Check sheet for the modelled part. Datum: model origin and axes. Units: mm. Face numbers are marked on the shaded views. A direction names the side the tool comes from. Give positions to 0.01 mm unless a question says otherwise; leave off trailing zeros. Write each loop counter-clockwise with the first axis right and the second up, starting at its lowest first coordinate (ties: lowest second). Pieces come first, ordered by that corner, then holes. Notation, with made-up numbers: (85, 63.25) -> (113, 63.25) arc R24 cw to (113, 88.25) -> close; hole circle Ø8 at (60.5, -9). An arc over 180 degrees is marked (long way). Answer as a JSON object with one key per item and string values.
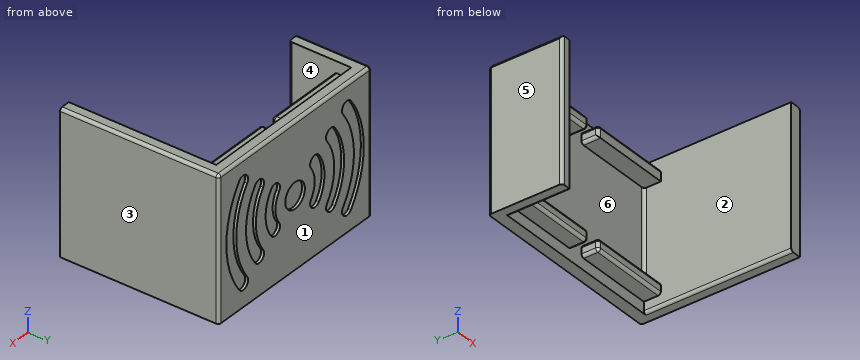
from build123d import *

# Parameters (mm, degrees)
SKETCH1_W           = 35
SKETCH1_H           = 25
BOSS_EXTRUDE1_DEPTH = 2
SKETCH3_W           = 2
SKETCH3_H           = 25
BOSS_EXTRUDE3_DEPTH = 11
SKETCH4_W           = 2
SKETCH4_H           = 25
BOSS_EXTRUDE4_DEPTH = 26
SKETCH5_W           = 14.3
SKETCH5_H           = 2
BOSS_EXTRUDE5_DEPTH = 3
SKETCH6_R           = 2.25
CUT_EXTRUDE1_DEPTH  = 0.5
FILLET1_R           = 0.5


with BuildPart() as part:
    # Sketch1 → Boss-Extrude1 (new body)
    with BuildSketch(Plane(origin=(0, 0, 0), x_dir=(1, 0, 0), z_dir=(0, 1, 0))):
        Rectangle(SKETCH1_W, SKETCH1_H)
    extrude(amount=BOSS_EXTRUDE1_DEPTH)

    # Sketch3 → Boss-Extrude3 (add)
    with BuildSketch(Plane(origin=(0, 0, 0), x_dir=(-1, 0, 0), z_dir=(0, -1, 0))):
        with Locations((16.5, 0)):
            Rectangle(SKETCH3_W, SKETCH3_H)
    extrude(amount=BOSS_EXTRUDE3_DEPTH)

    # Sketch4 → Boss-Extrude4 (add)
    with BuildSketch(Plane.XZ):
        with Locations((16.5, 0)):
            Rectangle(SKETCH4_W, SKETCH4_H)
    extrude(amount=BOSS_EXTRUDE4_DEPTH)

    # Sketch5 → Boss-Extrude5 (add)
    with BuildSketch(Plane.XZ):
        with Locations((8.35, 9.5)):
            Rectangle(SKETCH5_W, SKETCH5_H)
        with Locations((-8.35, 9.5)):
            Rectangle(SKETCH5_W, SKETCH5_H)
        with Locations((-8.35, -9.5)):
            Rectangle(SKETCH5_W, SKETCH5_H)
        with Locations((8.35, -9.5)):
            Rectangle(SKETCH5_W, SKETCH5_H)
    extrude(amount=BOSS_EXTRUDE5_DEPTH)

    # Sketch6 → Cut-Extrude1 (cut)
    with BuildSketch(Plane(origin=(0, 2, 0), x_dir=(1, 0, 0), z_dir=(0, 1, 0))):
        with Locations(Location((0, 0, 0), (0, 0, 270))):
            Circle(SKETCH6_R)
        with BuildLine():
            ThreePointArc((9.154501609, -6.538929598), (11.25, 1e-08), (9.154501598, 6.538929614))
            ThreePointArc((9.154501598, 6.538929614), (7.585158455, 6.800486886), (7.323601248, 5.231143733))
            ThreePointArc((7.323601248, 5.231143733), (9, -9e-09), (7.323601238, -5.231143747))
            ThreePointArc((7.323601238, -5.231143747), (7.58515847, -6.800486897), (9.154501609, -6.538929598))
        make_face()
        with BuildLine():
            ThreePointArc((-7.323601248, -5.231143733), (-9, -5e-09), (-7.323601254, 5.231143725))
            ThreePointArc((-7.323601254, 5.231143725), (-7.585158451, 6.800486883), (-9.154501598, 6.538929614))
            ThreePointArc((-9.154501598, 6.538929614), (-11.25, -1.2e-08), (-9.154501584, -6.538929633))
            ThreePointArc((-9.154501584, -6.538929633), (-7.585158446, -6.800486879), (-7.323601248, -5.231143733))
        make_face()
        with BuildLine():
            ThreePointArc((5.492700959, -3.923357768), (6.75, -1e-08), (5.492700971, 3.923357752))
            ThreePointArc((5.492700971, 3.923357752), (3.923357826, 4.184915008), (3.661800635, 2.615571852))
            ThreePointArc((3.661800635, 2.615571852), (4.5, -2.4e-08), (3.661800607, -2.61557189))
            ThreePointArc((3.661800607, -2.61557189), (3.923357837, -4.184915016), (5.492700959, -3.923357768))
        make_face()
        with BuildLine():
            ThreePointArc((-3.661800619, -2.615571874), (-4.5, 1.3e-08), (-3.661800604, 2.615571895))
            ThreePointArc((-3.661800604, 2.615571895), (-3.923357847, 4.184915023), (-5.492700971, 3.923357752))
            ThreePointArc((-5.492700971, 3.923357752), (-6.75, 0), (-5.492700971, -3.923357752))
            ThreePointArc((-5.492700971, -3.923357752), (-3.923357837, -4.184915016), (-3.661800619, -2.615571874))
        make_face()
        with BuildLine():
            ThreePointArc((10.985401866, 7.846715609), (13.5, 1.4e-08), (10.985401882, -7.846715586))
            ThreePointArc((10.985401882, -7.846715586), (11.246959012, -9.416058712), (12.81630214, -9.154501596))
            ThreePointArc((12.81630214, -9.154501596), (15.75, 2.5e-08), (12.816302111, 9.154501636))
            ThreePointArc((12.816302111, 9.154501636), (11.246959003, 9.416058706), (10.985401866, 7.846715609))
        make_face()
        with BuildLine():
            ThreePointArc((-10.985401876, -7.846715595), (-13.5, 4e-08), (-10.985401829, 7.84671566))
            ThreePointArc((-10.985401829, 7.84671566), (-11.246959061, 9.416058747), (-12.816302157, 9.154501571))
            ThreePointArc((-12.816302157, 9.154501571), (-15.75, 4.9e-08), (-12.816302215, -9.154501491))
            ThreePointArc((-12.816302215, -9.154501491), (-11.246959069, -9.416058753), (-10.985401876, -7.846715595))
        make_face()
    extrude(amount=-CUT_EXTRUDE1_DEPTH, mode=Mode.SUBTRACT)

    # Fillet1
    fillet1_edges = [part.edges().sort_by_distance(p)[0] for p in [
        (-17.5, 2, 0),
        (-17.5, -4.5, 12.5),
        (-17.5, -11, 0),
        (17.5, 2, 0),
        (17.5, -12, 12.5),
        (15.5, 0, 0),
        (-15.5, 0, 0),
        (8.35, -3, -8.5),
        (-8.35, -3, -8.5),
        (-8.35, -3, 8.5),
        (-8.35, -3, 10.5),
        (8.35, -3, 10.5),
        (-1.2, -1.5, 10.5),
        (-1.2, -1.5, 8.5),
        (1.2, -3, 9.5),
        (1.2, -1.5, 10.5),
        (1.2, -1.5, 8.5),
        (-1.2, -1.5, -10.5),
        (-1.2, -1.5, -8.5),
        (1.2, -1.5, -8.5),
        (1.2, -1.5, -10.5),
        (8.35, -3, -10.5),
        (-8.35, -3, -10.5),
        (0, 2, 12.5),
        (-15.5, -11, 0),
        (-1.2, -3, 9.5),
        (-1.2, -3, -9.5),
        (1.2, -3, -9.5),
        (15.5, -13, -12.5),
        (-15.5, -5.5, -12.5),
    ]]
    fillet(fillet1_edges, radius=FILLET1_R)


solid = part.part
1. Scan lines: L1, parallel to X at y = -9.25, z = 6.5; L2, parallel to Z at x = 14, y = -0.5; L3, parallel to Y at x = -9.5, z = 7. Record each from-to range of solid material in increasing order. Write a range as [from, to].
Determined:
{"L1": "[-17.5, -15.5], [15.5, 17.5]", "L2": "[-10.5, -8.5], [8.5, 10.5]", "L3": "[0, 2]"}
2. Go/stop test with flat-tipped pins: P1, Ø2.5, axis at x = 0, z = 0, coming from the -Y side; P2, Ø2, axis at x = -5.5, y = -1.5, coming from the +Z side; P3, Ø3, axis at x = -10.5, y = -1, coming from the -Z side; P4, Ø0.8, axis at x = -11.5, z = -9.5, coming from the -Y side. Record where each tip stops, or that it passes through.
Determined:
{"P1": "y = 0", "P2": "z = 10.5", "P3": "z = -12.5", "P4": "y = -3"}
3. Access from +Z, -Z, +X, -X, +Y, -Y to the whole of each face (thin tool, end or side, straight path). Record for the marked faces 5 and 6.
Determined:
{"face 5": "+Z, -Z, -X, +Y, -Y", "face 6": "-Y"}
4. Sectioned sample at B-B, the plane x = 0. Enter the section's corners in (y, z).
Determined:
{"outline": "(0, -12.5) -> (2, -12.5) -> (2, -2.25) -> (1.5, -2.25) -> (1.5, 2.25) -> (2, 2.25) -> (2, 12) arc R0.5 ccw to (1.5, 12.5) -> (0, 12.5) -> close"}
5. Mould release check, pull along X, two halves, no side actions. Record for the marked faces 1, 2, 3 and 4: released by +X, released by -X, zero draft, split by the parting line, or undercut.
Determined:
{"face 1": "zero draft", "face 2": "undercut", "face 3": "released by +X", "face 4": "undercut"}
6. Sectioned sample at A-A, the plane y = -5. Enter the section's corners in (x, z), plus the area to 3 significant figures.
Determined:
{"outline": "(-17.5, -12.5) -> (-16, -12.5) arc R0.5 ccw to (-15.5, -12) -> (-15.5, 12.5) -> (-17, 12.5) arc R0.5 ccw to (-17.5, 12) -> close; (15.5, -12) arc R0.5 ccw to (16, -12.5) -> (17.5, -12.5) -> (17.5, 12) arc R0.5 ccw to (17, 12.5) -> (15.5, 12.5) -> close", "area": "99.8 mm^2"}
7. Sectioned sample at D-D, the plane y = -14.5. Enter the section's corners in (x, z).
Determined:
{"outline": "(15.5, -12) arc R0.5 ccw to (16, -12.5) -> (17.5, -12.5) -> (17.5, 12) arc R0.5 ccw to (17, 12.5) -> (15.5, 12.5) -> close"}
